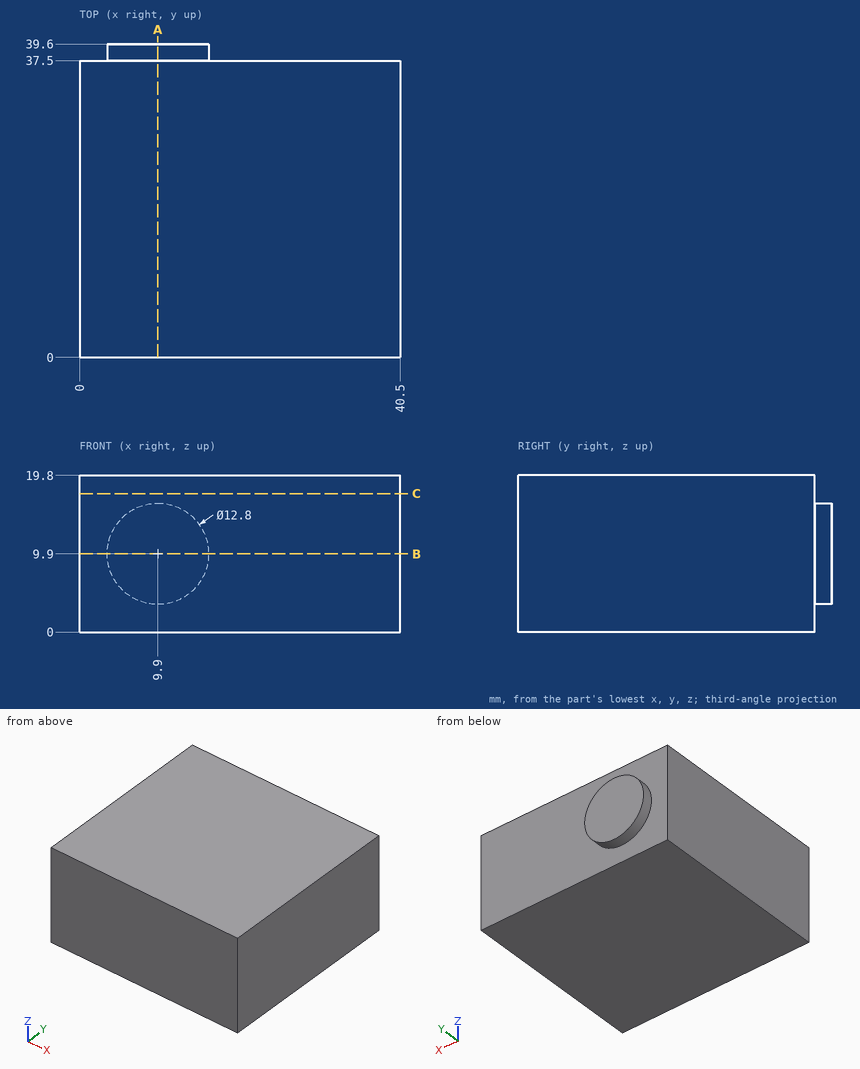
For this review, use the dimensioned drawing (mm, ordinates from the lowest corner) and the shaded views. Round coordinates to 2 decimals unless told otherwise and drop trailing zeros. Order: outer loops, then holes, each group sorted by start corner. A loop starts at its lowest first (then second) coordinate and runs counter-clockwise, first axis right, second up. Notation, with made-up numbers: (-11.75, 5) -> (26.25, 5) arc R15 ccw to (26.25, 33) -> close; hole circle Ø9 at (36.25, 0.25). An arc over 180 degrees is marked (long way). Write item = value, one per line. Start each with the question number.
Item 1: Consider section C-C on z = 17.5. Write out the cut boundary in (x, y).
Item 2: Consider section B-B on z = 9.9. Write out the cut boundary in (x, y), plus the area to 3 significant figures.
Item 3: Clearance check with a flat-ended pin moving along its axis: pin 1 Ø10 at (x, z) = (25.5, 7.5) entering from +Y. State where the tip first meets the part, or that it passes through.
Item 4: For line 1 along Y through (x, z) = (10, 3.25), list the stretches that pass through material, from the lowest coordinate up.
Item 5: Consider section A-A on x = 9.9. Write out the cut boundary in (y, z).
Conclusion:
q1.outline = (0, 0) -> (40.5, 0) -> (40.5, 37.5) -> (0, 37.5) -> close
q2.outline = (0, 0) -> (40.5, 0) -> (40.5, 37.5) -> (16.3, 37.5) -> (16.3, 39.6) -> (3.5, 39.6) -> (3.5, 37.5) -> (0, 37.5) -> close
q2.area = 1,550 mm2
q3.pin_1 = 37.5
q4.line_1 = 0 to 37.5
q5.outline = (0, 0) -> (37.5, 0) -> (37.5, 3.5) -> (39.6, 3.5) -> (39.6, 16.3) -> (37.5, 16.3) -> (37.5, 19.8) -> (0, 19.8) -> close
